```python
from build123d import *

# Parameters (mm, degrees)
F0_W     = 380
F0_H     = 380
F1_DEPTH = 350
F2_W     = 361
F2_H     = 331
F3_DEPTH = 361
F4_W     = 40
F4_H     = 40
F5_DEPTH = 100
F6_W     = 40
F6_H     = 40
F7_DEPTH = 100


with BuildPart() as f1:
    # F0 (on Top) → F1 (new body)
    with BuildSketch(Plane.XY):
        Rectangle(F0_W, F0_H)
    extrude(amount=F1_DEPTH)

    # F2 (on face) → F3 (cut)
    with BuildSketch(Plane.XZ.offset(190)):
        with Locations((0, 175)):
            Rectangle(F2_W, F2_H)
    extrude(amount=-F3_DEPTH, mode=Mode.SUBTRACT)

    # F4 (on face) → F5 (join)
    with BuildSketch(Plane.XY.offset(350)):
        with Locations((-170, 170)):
            Rectangle(F4_W, F4_H)
        with Locations((170, 170)):
            Rectangle(F4_W, F4_H)
    extrude(amount=F5_DEPTH)

    # F6 (on face) → F7 (join)
    with BuildSketch(Plane.XY.offset(350)):
        with Locations((-170, -170)):
            Rectangle(F6_W, F6_H)
        with Locations((170, -170)):
            Rectangle(F6_W, F6_H)
    extrude(amount=F7_DEPTH)


solid = f1.part
```
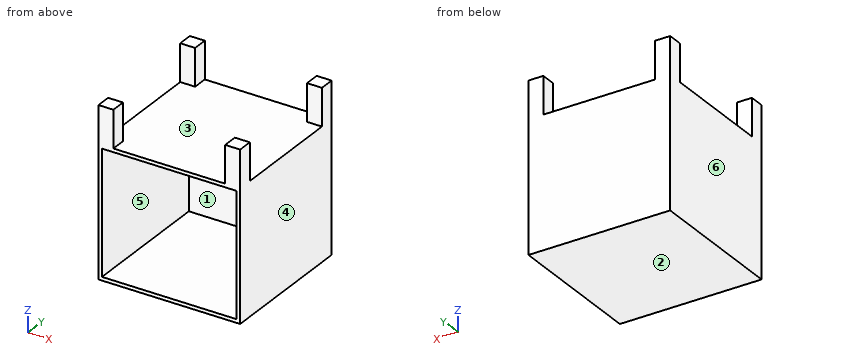
CAD build for the part. Positions are in the model's coordinates, mm. Face numbers are marked on the shaded views. A direction names the side the tool comes from. Give positions to 0.01 mm unless a question says otherwise; leave off trailing zeros. Order: outer loops, then holes, each group sorted by start corner. A loop starts at its lowest first (then second) coordinate and runs counter-clockwise, first axis right, second up.
(1) Saw through at B-B, the plane z = 356.5. Give the cut face in (x, y).
(2) Tool access for the marked faces 1 and 2: list every direction of +Z, -Z, +X, -X, +Y, -Y with a clear straight run to the whole face (end or side of a thin tool).
(3) Mould opens along X. For the marked faces 3, 4, 5 and 6 say: released by +X, released by -X, zero draft, split by the parting line, or undercut.
(4) Drill centre lines: L1, parallel to Z at x = -114, y = 62; L2, parallel to X at y = 39.5, z = 40; L3, parallel to Y at x = -97.5, z = 216. Where is each one in solid material? Low to high.
(5) Saw through at D-D, the plane z = 167.5. Give the cut face in (x, y).
(6) Saw through at A-A, the plane y = 70. Give the cut face in (x, z), then the cut area to 3 significant figures.
(7) Flat gauge pins, fed straight in: pin 1 (10 mm diameter, centred on x = 77.5, y = 133, fed in from +Z); pin 2 (1 mm diameter, centred on x = 132.5, z = 325.5, fed in from -Y). Where does each tip first touch, or does it go through?
(8) Saw through at C-C, the plane x = 37.5. Give the cut face in (y, z), then the cut area to 3 significant figures.
Results found:
1. outline: (-190, -190) - (-150, -190) - (-150, -150) - (-190, -150) - close; (-190, 150) - (-150, 150) - (-150, 190) - (-190, 190) - close; (150, -190) - (190, -190) - (190, -150) - (150, -150) - close; (150, 150) - (190, 150) - (190, 190) - (150, 190) - close
2. face 1: -Y
2. face 2: -Z, +X, -X, +Y, -Y
3. face 3: undercut
3. face 4: released by +X
3. face 5: undercut
3. face 6: released by -X
4. L1: z = 0 to 9.5, 340.5 to 350
4. L2: x = -190 to -180.5, 180.5 to 190
4. L3: y = 171 to 190
5. outline: (-190, -190) - (-180.5, -190) - (-180.5, 171) - (180.5, 171) - (180.5, -190) - (190, -190) - (190, 190) - (-190, 190) - close
6. outline: (-190, 0) - (190, 0) - (190, 350) - (-190, 350) - close; hole (-180.5, 9.5) - (180.5, 9.5) - (180.5, 340.5) - (-180.5, 340.5) - close
6. area: 13,500 mm2
7. pin 1: stops at z = 350
7. pin 2: stops at y = 171
8. outline: (-190, 0) - (190, 0) - (190, 350) - (-190, 350) - (-190, 340.5) - (171, 340.5) - (171, 9.5) - (-190, 9.5) - close
8. area: 13,500 mm2
